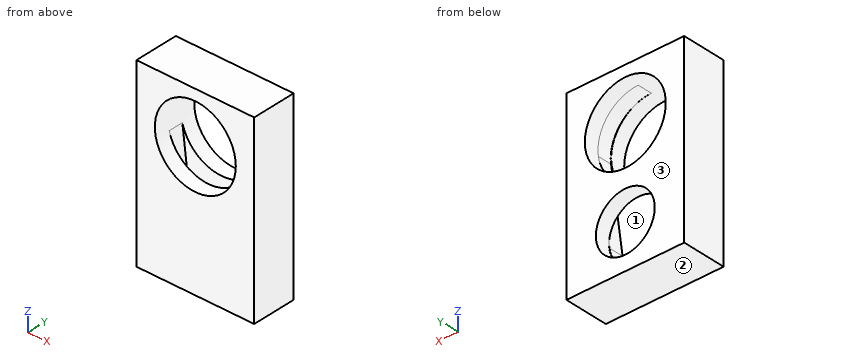
from build123d import *

# Parameters (mm, degrees)
F2_W     = 80
F2_H     = 125
F2_R     = 27.5
F3_DEPTH = 30
F4_START = 10
F4_DEPTH = 10
F1_R     = 20
F5_DEPTH = 10


with BuildPart() as f3:
    # F2 (on Front) → F3 (new body)
    with BuildSketch(Plane.XZ):
        with Locations((0, 12.5)):
            Rectangle(F2_W, F2_H)
        with Locations((0, 40)):
            Circle(F2_R, mode=Mode.SUBTRACT)
    extrude(amount=F3_DEPTH)

    # F0 (on Front) → F4 (cut)
    with BuildSketch(Plane.XZ.offset(F4_START)):
        with BuildLine():
            ThreePointArc((27.5, 36.3901084755), (0.4118554049, 67.4994501998), (-27.0675471314, 36.7351664218))
            Line((-27.0675471314, 36.7351664218), (-20, -22.3744244205))
            ThreePointArc((-20, -22.3744244205), (-0.2679149621, -39.9996001453), (19.6854888228, -22.6253756542))
            Line((19.6854888228, -22.6253756542), (27.5, 36.3901084755))
        make_face()
    extrude(amount=F4_DEPTH, mode=Mode.SUBTRACT)

    # F1 (on Front) → F5 (cut)
    with BuildSketch(Plane.XZ):
        with Locations((0, -20)):
            Circle(F1_R)
    extrude(amount=F5_DEPTH, mode=Mode.SUBTRACT)


solid = f3.part
Geometry check sheet. Reference: the model listing, model coordinates, mm. Face numbers are marked on the shaded views. Give positions to 0.01 mm unless a question says otherwise; leave off trailing zeros. Loops run counter-clockwise (first coordinate to the right, second up) from the corner with the lowest first, then second, coordinate; pieces in that order, holes last. Notation, with made-up numbers: M 37,26.5 L 92,26.5 A29 ccw 92,52.5 Z; hole C -25,40 d5. An arc over 180 degrees is marked long. Write each question's results on one line, items separated by ' | '.
1) Release check for a two-part mould opening along Y. For the marked faces 1, 2 and 3 record: +Y half, -Y half, draft (parallel to the pull), parting line (faces both ways), or undercut.
Answers follow:
face 1: undercut | face 2: draft | face 3: +Y half
2) Section check C-C, the plane x = -17.5. Record the boundary of the cut face in (y, z), plus the area to 3 significant figures.
Answers follow:
outline: M -30,-50 L 0,-50 L 0,-29.68 L -10,-29.68 L -10,-29.93 L -20,-29.93 L -20,18.79 L -30,18.79 Z; M -30,61.21 L 0,61.21 L 0,75 L -30,75 Z; M -10,-10.32 L 0,-10.32 L 0,18.79 L -10,18.79 Z | area: 1,800 mm2
3) Section check B-B, the plane y = -27. Record the boundary of the cut face in (x, z), plus the area to 3 significant figures.
Answers follow:
outline: M -40,-50 L 40,-50 L 40,75 L -40,75 Z; hole C 0,40 d55 | area: 7,620 mm2
4) Section check A-A, the plane z = 40. Record the boundary of the cut face in (x, y), plus the area to 3 significant figures.
Answers follow:
outline: M -40,-30 L -27.5,-30 L -27.5,0 L -40,0 Z; M 27.5,-30 L 40,-30 L 40,0 L 27.5,0 L 27.5,-10 L 27.74,-10 L 27.74,-20 L 27.5,-20 Z | area: 748 mm2
5) Thickness scan on line 1 (Z direction, x = 0, y = -2.5); line 2 (Y direction, x = -18, z = 5); line 3 (Z direction, x = 0, y = -15.25). Record the ranges inside material, lowest first.
Answers follow:
line 1: -50 to -40, 0 to 12.5, 67.5 to 75 | line 2: -30 to -20, -10 to 0 | line 3: -50 to -40, 67.5 to 75
6) Gauge pin test, flat end, axial feed: pin 1 (4 mm diameter, centred on x = -29.5, z = -33.5, fed in from +Y). Record the tip position at first contact, or that the pin passes through.
Answers follow:
pin 1: y = 0
7) Section check D-D, the plane y = -5. Record the boundary of the cut face in (x, z).
Answers follow:
outline: M -40,-50 L 40,-50 L 40,75 L -40,75 Z; hole C 0,40 d55; hole C 0,-20 d40
